Build history of the part. All positions in model axes, mm. Face numbers are marked on the shaded views. A direction names the side the tool comes from. Coordinates: 2 decimals unless noted, no trailing zeros. Order: outer loops, then holes, each group sorted by start corner. A loop starts at its lowest first (then second) coordinate and runs counter-clockwise, first axis right, second up. Notation, with made-up numbers: (10, -13.75) - (40, -13.75) arc R23 cw to (40, 20.25) - close; hole circle Ø10 at (51.5, 16). An arc over 180 degrees is marked (long way). Write each question's results on one line, items separated by ' | '.
Autodesk Inventor part; units mm, degrees
ref_plane "YZ Plane" through (0, 0, 0) normal (1, 0, 0) x (0, 1, 0)
ref_plane "XZ Plane" through (0, 0, 0) normal (0, 1, 0) x (-1, 0, 0)
ref_plane "XY Plane" through (0, 0, 0) normal (0, 0, 1) x (1, 0, 0)
sketch "草圖1" plane through (0, 0, 0) normal (0, 0, 1) x (1, 0, 0)
  circle A0 centre (0, 0) radius 11.725
  dimension "d0" = 23.45
extrude "擠出1" add sketch "草圖1" along normal blind 7.9
sketch "草圖2" plane through (0, 0, 7.9) normal (0, 0, 1) x (1, 0, 0)
  circle A0 centre (0, 0) radius 5
  dimension "d3" = 10
extrude "擠出2" add sketch "草圖2" along normal blind 6.3
hole "孔1" at (0, 0, 14.2) direction (0, 0, -1) diameter 6 end through all
chamfer "倒角1" distance 0.5 angle 45 3 edges at (0, 3, 14.2) (0, 3, 0) (-5, 0, 14.2)
sketch "草圖3" plane through (0, 0, 0) normal (1, 0, 0) x (0, 1, 0)
  circle A0 centre (0, 10.9) radius 1.175
  line L0 (-4.5, 14.2) -> (4.5, 14.2)
  point P0 (0, 0)
  dimension "d18" = 2.35
  dimension "d19" = 3.3
extrude "擠出3" cut sketch "草圖3" against normal through all
properties part number "齒輪"
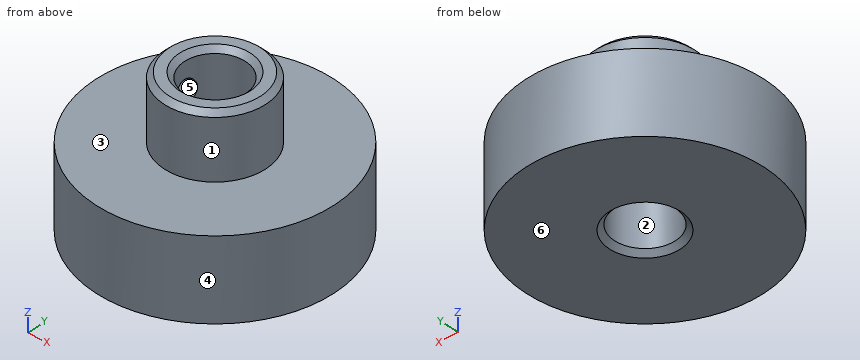
1. Two-plate mould, pull along Z, no slides. Class the marked faces 3, 4, 5 and 6: +Z half, -Z half, draft (parallel to the pull), parting line (faces both ways), or undercut.
Solved:
face 3: +Z half | face 4: draft | face 5: undercut | face 6: -Z half
2. Band-saw the part on B-B on x = 0. Give the cut face in (y, z) (3 decimals), then the cut area to 3 significant figures.
Solved:
outline: (-11.725, 0) - (-3.5, 0) - (-3, 0.5) - (-3, 13.7) - (-3.5, 14.2) - (-4.5, 14.2) - (-5, 13.7) - (-5, 7.9) - (-11.725, 7.9) - close; (3, 0.5) - (3.5, 0) - (11.725, 0) - (11.725, 7.9) - (5, 7.9) - (5, 13.7) - (4.5, 14.2) - (3.5, 14.2) - (3, 13.7) - close | area: 162 mm2
3. Tool access for the marked faces 1 and 2: list every direction of +Z, -Z, +X, -X, +Y, -Y with a clear straight run to the whole face (end or side of a thin tool).
Solved:
face 1: +Z | face 2: +Z, -Z
4. Band-saw the part on A-A on y = 0. Give the cut face in (x, z) (3 decimals), then the cut area to 3 significant figures.
Solved:
outline: (-11.725, 0) - (-3.5, 0) - (-3, 0.5) - (-3, 9.725) - (-5, 9.725) - (-5, 7.9) - (-11.725, 7.9) - close; (-5, 12.075) - (-3, 12.075) - (-3, 13.7) - (-3.5, 14.2) - (-4.5, 14.2) - (-5, 13.7) - close; (3, 0.5) - (3.5, 0) - (11.725, 0) - (11.725, 7.9) - (5, 7.9) - (5, 13.7) - (4.5, 14.2) - (3.5, 14.2) - (3, 13.7) - close | area: 158 mm2
5. Band-saw the part on C-C on z = 6.5. Give the cut face in (x, y) (3 decimals).
Solved:
outline: circle Ø23.45 at (0, 0); hole circle Ø6 at (0, 0)
6. Probe line 1 (Y direction, x = 0, z = 8.5); line 2 (Z direction, x = -6.5, y = -4); line 3 (X direction, y = 0.5, z = 13.25). List the from-to ranges inside material, lowest first.
Solved:
line 1: y = -5 to -3, 3 to 5 | line 2: z = 0 to 7.9 | line 3: x = -4.97 to -2.96, 2.96 to 4.97
7. Band-saw the part on D-D on y = -8.25. Give the cut face in (x, z).
Solved:
outline: (-8.33, 0) - (8.33, 0) - (8.33, 7.9) - (-8.33, 7.9) - close
8. Drop flat-ended pins along their axis: pin 1 Ø8 at (x, z) = (8, 9) entering from +Y; pin 2 Ø4 at (x, y) = (8.5, 7.5) entering from +Z; pin 3 Ø3 at (y, z) = (-3, 11.5) entering from -X. Give the stop position or say it passes through.
Solved:
pin 1: stops at y = 10.96 | pin 2: stops at z = 7.9 | pin 3: stops at x = -4.77
